Input: part model. Units: mm. Frame: model coordinates. A direction names the side the tool comes from. Coordinates: 2 decimals unless noted, no trailing zeros. Order: outer loops, then holes, each group sorted by start corner. A loop starts at its lowest first (then second) coordinate and runs counter-clockwise, first axis right, second up. Notation, with made-up numbers: (50.5, 5) -> (60.5, 5) arc R35 cw to (60.5, 40) -> close; hole circle Ø5 at (45.5, 43). An arc over 180 degrees is marked (long way). Use one line per item in the form item = value. Start each with the question number.
1) Ray query, line 1 along X through (y, z) = (16.5, -28); line 2 along Z through (x, y) = (-169.5, 3); line 3 along X through (y, z) = (-3.5, -64). Return the intervals inside material, ascending.
2) Pin query (flat end, axial travel): pin 1 (10 mm diameter, centred on y = 15, z = -13.5, fed in from +X); pin 2 (3 mm diameter, centred on y = 146.5, z = 67, fed in from -X); pin 3 (2.5 mm diameter, centred on x = -197, y = 0, fed in from +Z). Return the tip coordinate at first contact, or that it passes through.
3) Access query for faces 1 (the flat face through (-50.42, 146.68, 65.47)), 2 (the cylindrical face through (-146.84, 14.66, -64.23)), 3 (the cylindrical face through (-90.14, 146.69, 66.902)), 4 (the flat face through (-1.4, -5.07, 13.53)). Directions: +Z, -Z, +X, -X, +Y, -Y. A direction counts if a zero-diameter tool reaches every point of the face in a straight line with its end or side. Return the directions, or none.
4) Section query A-A on z = -25. Output: boundary loops of the cut face in (x, y), then the cut area to 3 significant figures.
5) Section query C-C on x = -16. Output: boundary loops of the cut face in (y, z), then the cut area to 3 significant figures.
6) Draft query along Z for faces 5 (the flat face through (-92, 10, -40)), 6 (the flat face through (-165, 29.559, -64)), 7 (the flat face through (-147, -8, -65)), 8 (the flat face through (-96, 29.559, -38)). Return one class per face: pulls with the +Z half, pulls with the -Z half, needs draft (parallel to the pull), parting line crosses it, or undercut.
7) Section query B-B on y = 42.5. Output: boundary loops of the cut face in (x, z), then the cut area to 3 significant figures.
8) Section query D-D on z = 14. Output: boundary loops of the cut face in (x, y).
from build123d import *

# Parameters (mm, degrees)
SKETCH1_W                = 200
SKETCH1_H                = 150
BOSS_EXTRUDE1_DEPTH      = 15
SKETCH1_5_W              = 200
SKETCH1_5_H              = 10
REVOLVE1_ANGLE           = 90
BOSS_EXTRUDE3_REACH      = 197.256
BOSS_EXTRUDE3_END_RADIUS = 140
SKETCH1_6_W              = 10
SKETCH1_6_H              = 10
CUT_EXTRUDE2_DEPTH       = 60
CUT_EXTRUDE3_DEPTH       = 20
CUT_LOFT8_START          = -65
CUT_LOFT8_DEPTH          = 130
CUT_LOFT8_START_2        = -100
CUT_LOFT8_2_DEPTH        = 200
BOSS_EXTRUDE5_DEPTH      = 100
BOSS_EXTRUDE6_START      = -8
BOSS_EXTRUDE6_DEPTH      = 8
BOSS_EXTRUDE7_START      = -5
BOSS_EXTRUDE7_DEPTH      = 5


with BuildPart() as part:
    # Sketch1 → Boss-Extrude1 (new body)
    with BuildSketch(Plane(origin=(0, 0, 0), x_dir=(1, 0, 0), z_dir=(0, 1, 0))):
        Rectangle(SKETCH1_W, SKETCH1_H)
    extrude(amount=-BOSS_EXTRUDE1_DEPTH)

    # Sketch1<5> → Revolve1 (revolve)
    with BuildSketch(Plane(origin=(0, 0, 0), x_dir=(1, 0, 0), z_dir=(0, 1, 0))):
        with Locations((0, 70)):
            Rectangle(SKETCH1_5_W, SKETCH1_5_H)
    revolve(axis=Axis((-100, 0, 75), (1, 0, 0)), revolution_arc=REVOLVE1_ANGLE)

    # Boss-Extrude3: up to this cylinder (the profile starts inside it)
    boss_extrude3_end = Plane(origin=(0, 0, 75), z_dir=(-1, 0, 0)) * Cylinder(BOSS_EXTRUDE3_END_RADIUS, 865.512, mode=Mode.PRIVATE)
    # Sketch1<6> → Boss-Extrude3 (add, up to the surface)
    with BuildSketch(Plane(origin=(0, 0, 0), x_dir=(1, 0, 0), z_dir=(0, 1, 0)), mode=Mode.PRIVATE) as boss_extrude3_sk1:
        with Locations((-95, -70)):
            Rectangle(SKETCH1_6_W, SKETCH1_6_H)
    boss_extrude3_tool1 = extrude(boss_extrude3_sk1.sketch, amount=BOSS_EXTRUDE3_REACH, mode=Mode.PRIVATE) & boss_extrude3_end
    add(boss_extrude3_tool1.solids().sort_by_distance((-95, 0, 70))[0])
    # Sketch1<6> → Boss-Extrude3 (add, up to the surface)
    with BuildSketch(Plane(origin=(0, 0, 0), x_dir=(1, 0, 0), z_dir=(0, 1, 0)), mode=Mode.PRIVATE) as boss_extrude3_sk2:
        with Locations((95, -70)):
            Rectangle(SKETCH1_6_W, SKETCH1_6_H)
    boss_extrude3_tool2 = extrude(boss_extrude3_sk2.sketch, amount=BOSS_EXTRUDE3_REACH, mode=Mode.PRIVATE) & boss_extrude3_end
    add(boss_extrude3_tool2.solids().sort_by_distance((95, 0, 70))[0])

    # Sketch5 → Cut-Extrude2 (cut)
    with BuildSketch(Plane.ZY.offset(80)):
        Polygon((66.095917942, 143.620915339), (26.904082058, 135.620915339), (21.904082058, 160.115812766), (61.095917942, 168.115812766), align=None)
    extrude(amount=-CUT_EXTRUDE2_DEPTH, mode=Mode.SUBTRACT)

    # Sketch6 → Cut-Extrude3 (cut)
    with BuildSketch(Plane.ZY.offset(100)):
        with BuildLine():
            Line((55, 144.203533404), (65, 144.203533404))
            ThreePointArc((65, 144.203533404), (60, 157.655), (55, 144.203533404))
        make_face()
    extrude(amount=-CUT_EXTRUDE3_DEPTH, mode=Mode.SUBTRACT)

    # Cut-Loft8: read off the stored shape, not the designer's step
    # Cut-Loft8 outline → Cut-Loft8 (cut)
    with BuildSketch(Plane.XY.offset(CUT_LOFT8_START)):
        Polygon((-100, -10), (100, 0), (-100, 0), align=None)
    extrude(amount=CUT_LOFT8_DEPTH, mode=Mode.SUBTRACT)

    # Cut-Loft8 2 outline → Cut-Loft8 2 (add)
    with BuildSketch(Plane.YZ.offset(CUT_LOFT8_START_2)):
        Polygon((0, -65), (-10.4, -13), (-12, -13), (-12, -65), align=None)
    extrude(amount=CUT_LOFT8_2_DEPTH)

    # Sketch12 → Boss-Extrude5 (add)
    with BuildSketch(Plane.ZY.offset(100)):
        with BuildLine():
            Line((-65, -15), (-65, 0))
            ThreePointArc((-65, 0), (-64.208776017, 14.863266125), (-61.84404743, 29.558529783))
            Line((-61.84404743, 29.558529783), (-72.058809043, 29.558529783))
            ThreePointArc((-72.058809043, 29.558529783), (-74.262891163, 14.852249722), (-75, 0))
            Line((-75, 0), (-75, -15))
            Line((-75, -15), (-65, -15))
        make_face()
    extrude(amount=BOSS_EXTRUDE5_DEPTH)

    # Sketch12<4> → Boss-Extrude6 (add)
    with BuildSketch(Plane.ZY.offset(100).offset(BOSS_EXTRUDE6_START)):
        with BuildLine():
            Line((-65, 0), (-15, -10))
            Line((-15, -10), (-15, 29.558529783))
            Line((-15, 29.558529783), (-61.84404743, 29.558529783))
            ThreePointArc((-61.84404743, 29.558529783), (-64.208776017, 14.863266125), (-65, 0))
        make_face()
    extrude(amount=BOSS_EXTRUDE6_DEPTH)

    # Sketch21 → Boss-Extrude7 (add)
    with BuildSketch(Plane.ZY.offset(200).offset(BOSS_EXTRUDE7_START)):
        with BuildLine():
            Line((-61.84404743, 29.558529783), (72.644533384, 29.558529783))
            Line((72.644533384, 29.558529783), (72.644533384, -15))
            Line((72.644533384, -15), (-65, -15))
            Line((-65, -15), (-65, 0))
            ThreePointArc((-65, 0), (-64.208776017, 14.863266125), (-61.84404743, 29.558529783))
        make_face()
    extrude(amount=BOSS_EXTRUDE7_DEPTH)


solid = part.part
Answers below:
q1.line_1 = -200 to -195, -100 to -92
q1.line_2 = -74.97 to -64.97
q1.line_3 = -200 to -195, -100 to 100
q2.pin_1 = -92
q2.pin_2 = -100
q2.pin_3 = 72.64
q3.face_1 = -Z
q3.face_2 = +Z, -Y
q3.face_3 = -X, +Y
q3.face_4 = none
q4.outline = (-200, -15) -> (-195, -15) -> (-195, 29.56) -> (-200, 29.56) -> close; (-100, -15) -> (100, -15) -> (100, 0) -> (-60, -8) -> (-92, -8) -> (-92, 29.56) -> (-100, 29.56) -> close; (-100, 97.98) -> (100, 97.98) -> (100, 111.8) -> (-100, 111.8) -> close
q4.area = 5,330 mm^2
q5.outline = (-15, -75) -> (0, -75) arc R150 ccw to (150, 75) -> (140, 75) arc R140 cw to (0, -65) -> (-5.8, -36) -> (-5.8, 65) -> (0, 65) -> (0, 75) -> (-15, 75) -> close
q5.area = 3,860 mm^2
q6.face_5 = undercut
q6.face_6 = needs draft
q6.face_7 = pulls with the +Z half
q6.face_8 = undercut
q7.outline = (-100, -68.85) -> (100, -68.85) -> (100, -58.39) -> (-100, -58.39) -> close; (-100, 65) -> (-90, 65) -> (-90, 75) -> (-100, 75) -> close; (90, 65) -> (100, 65) -> (100, 75) -> (90, 75) -> close
q7.area = 2,290 mm^2
q8.outline = (-200, -15) -> (-195, -15) -> (-195, 29.56) -> (-200, 29.56) -> close; (-100, -15) -> (100, -15) -> (100, 0) -> (-100, -10) -> close; (-100, 126.01) -> (100, 126.01) -> (100, 137.04) -> (-100, 137.04) -> close
